Autodesk Inventor part; units mm, degrees
ref_plane "YZ Plane" through (0, 0, 0) normal (1, 0, 0) x (0, 1, 0)
ref_plane "XZ Plane" through (0, 0, 0) normal (0, 1, 0) x (-1, 0, 0)
ref_plane "XY Plane" through (0, 0, 0) normal (0, 0, 1) x (1, 0, 0)
sketch "Sketch1" plane through (0, 0, 0) normal (0, 1, 0) x (-1, 0, 0)
  circle A0 centre (0, 0) radius 50.8
  dimension "d0" = 101.6
extrude "Extrusion1" add sketch "Sketch1" along normal blind 5.588
sketch "Sketch2" plane through (0, 5.588, 0) normal (0, 1, 0) x (1, 0, 0)
  line L0 (3.81, 13.97) -> (-3.81, 13.97)
  line L1 (-3.81, 13.97) -> (-3.81, -13.97)
  line L2 (-3.81, -13.97) -> (3.81, -13.97)
  line L3 (3.81, -13.97) -> (3.81, 13.97)
  point P0 (0, 0)
  dimension "d3" = 7.62
  dimension "d4" = 27.94
extrude "Extrusion2" cut sketch "Sketch2" against normal blind 5.588
sketch "Sketch3" plane through (0, 5.588, 0) normal (0, 1, 0) x (1, 0, 0)
  point P0 (0, 0)
sketch "Sketch4" plane through (0, 5.588, 0) normal (0, 1, 0) x (1, 0, 0)
  line L0 (3.81, 15.24) -> (-3.81, 15.24)
  line L1 (-3.81, 15.24) -> (-3.81, -15.24)
  line L2 (-3.81, -15.24) -> (3.81, -15.24)
  line L3 (3.81, -15.24) -> (3.81, 15.24)
  point P0 (0, 0)
  dimension "d7" = 30.48
extrude "Extrusion3" cut sketch "Sketch4" against normal blind 5.588
sketch "Sketch5" plane through (0, 5.588, 0) normal (0, 1, 0) x (1, 0, 0)
  line L0 (3.81, 15.24) -> (-3.81, 15.24)
  circle A0 centre (0, 15.24) radius 3.81
  point P0 (0, 0)
  dimension "d10" = 7.62
extrude "Extrusion4" cut sketch "Sketch5" against normal blind 5.588
sketch "Sketch6" plane through (0, 5.588, 0) normal (0, 1, 0) x (1, 0, 0)
  line L0 (-3.81, -15.24) -> (3.81, -15.24)
  circle A0 centre (0, -15.24) radius 3.81
  point P0 (0, 0)
  dimension "d13" = 7.62
extrude "Extrusion5" cut sketch "Sketch6" against normal blind 5.588
sketch "Sketch7" plane through (0, 5.588, 0) normal (0, 1, 0) x (1, 0, 0)
  point P0 (0, 0)
properties part number "midCup"
The listing builds one solid part. Answer for the finished solid, in the listing's coordinates (mm). A direction names the side the tool comes from. Coordinates: 2 decimals unless noted, no trailing zeros. Write each loop counter-clockwise with the first axis right and the second up, starting at its lowest first coordinate (ties: lowest second). Pieces come first, ordered by that corner, then holes. Notation, with made-up numbers: (0, 38) - (28, 38) arc R26 cw to (28, 73) - close; hole circle Ø7 at (25, 62.5). An arc over 180 degrees is marked (long way). Return JSON: item names as keys, results as strings.
1. Consider line 1 along X through (y, z) = (2.3, 4); line 2 along X through (y, z) = (5, 11); line 3 along Z through (x, y) = (4, 4.4). Determine where each line is inside the solid, lowest interval first.
Final values:
{"line 1": "-50.64 to -3.81, 3.81 to 50.64", "line 2": "-49.59 to -3.81, 3.81 to 49.59", "line 3": "-50.64 to 50.64"}
2. The part is cut by section B-B on x = 0. Determine the outline of the cut face in (y, z), then the cut area to 3 significant figures.
Final values:
{"outline": "(0, -50.8) - (5.59, -50.8) - (5.59, -19.05) - (0, -19.05) - close; (0, 19.05) - (5.59, 19.05) - (5.59, 50.8) - (0, 50.8) - close", "area": "355 mm^2"}
3. Which of the six approach directions +Z, -Z, +X, -X, +Y, -Y give full straight-line access (tool end or side, diameter ignored) to faces 1 (the face through (-11, 0, 1)), 2 (the face through (-3.81, 3, 0))?
Final values:
{"face 1": "+Z, -Z, +X, -X, -Y", "face 2": "+Y, -Y"}
4. The part is cut by section A-A on z = 0. Determine the outline of the cut face in (x, y), then the cut area to 3 significant figures.
Final values:
{"outline": "(-50.8, 0) - (-3.81, 0) - (-3.81, 5.59) - (-50.8, 5.59) - close; (3.81, 0) - (50.8, 0) - (50.8, 5.59) - (3.81, 5.59) - close", "area": "525 mm^2"}
5. For a pull along Z with two mould halves and no side action, classify faces 3 (the face through (11.012, 2.755, 49.592)), 4 (the face through (-11, 5.588, 1)), 5 (the face through (0.08, 2.83, -19.05)) as +Z half, -Z half, draft (parallel to the pull), parting line (faces both ways), or undercut.
Final values:
{"face 3": "parting line", "face 4": "draft", "face 5": "undercut"}
6. The part is cut by section C-C on y = 3.15. Determine the outline of the cut face in (x, z), then the cut area to 3 significant figures.
Final values:
{"outline": "circle Ø101.6 at (0, 0); hole (-3.81, -15.24) arc R3.81 ccw to (3.81, -15.24) - (3.81, 15.24) arc R3.81 ccw to (-3.81, 15.24) - close", "area": "7,830 mm^2"}
7. Each of these flat-tipped pins is pushed along its axis until it touches: pin 1 Ø1 at (x, y) = (29.5, 4.5) entering from -Z; pin 2 Ø1.5 at (x, y) = (-37, 0.5) entering from -Z; pin 3 Ø1.5 at (x, y) = (-3, 3) entering from -Z. Where does it stop, or does it pass through?
Final values:
{"pin 1": "z = -41.71", "pin 2": "z = -35.59", "pin 3": "z = -50.75"}
8. The part is cut by section D-D on x = -26. Determine the outline of the cut face in (y, z).
Final values:
{"outline": "(0, -43.64) - (5.59, -43.64) - (5.59, 43.64) - (0, 43.64) - close"}
